For this review, use the dimensioned drawing (mm, ordinates from the lowest corner) and the shaded views. Round coordinates to 2 decimals unless told otherwise and drop trailing zeros. Order: outer loops, then holes, each group sorted by start corner. A loop starts at its lowest first (then second) coordinate and runs counter-clockwise, first axis right, second up. Notation, with made-up numbers: (84, -11) - (105, -11) arc R7 ccw to (105, -3) - close; hole circle Ø3 at (27.5, 76). An arc over 180 degrees is marked (long way). Write each question's results on one line, items separated by ' | '. Start each with the question number.
(1) Take a section at D-D, the plane y = 12.75. Give the boundary of the cut face in (x, z), plus the area to 3 significant figures.
(2) Take a section at B-B, the plane z = 27.5. Give the boundary of the cut face in (x, y).
(3) Take a section at A-A, the plane x = 28.5. Give the boundary of the cut face in (y, z), plus the area to 3 significant figures.
(4) For L1, parallel to X at y = 2.25, z = 28; L2, parallel to X at y = 10.75, z = 34; L3, parallel to Y at x = 28, z = 46, list the stretches that pass through material, from the lowest coordinate up. Write a range as from..to.
(5) Insertion check: pin 1 Ø9 at (x, y) = (28.5, 10) entering from +Z; pin 2 Ø2 at (x, y) = (43, 4) entering from -Z; pin 3 Ø1 at (y, z) = (6.5, 22) entering from -X; pin 4 Ø5 at (x, y) = (25.5, 18) entering from -Z. Each pin has a flat end and moves straight along its axis. Give the tip position at first contact, or say it passes through.
(6) Take a section at C-C, the plane y = 18. Give the boundary of the cut face in (x, z).
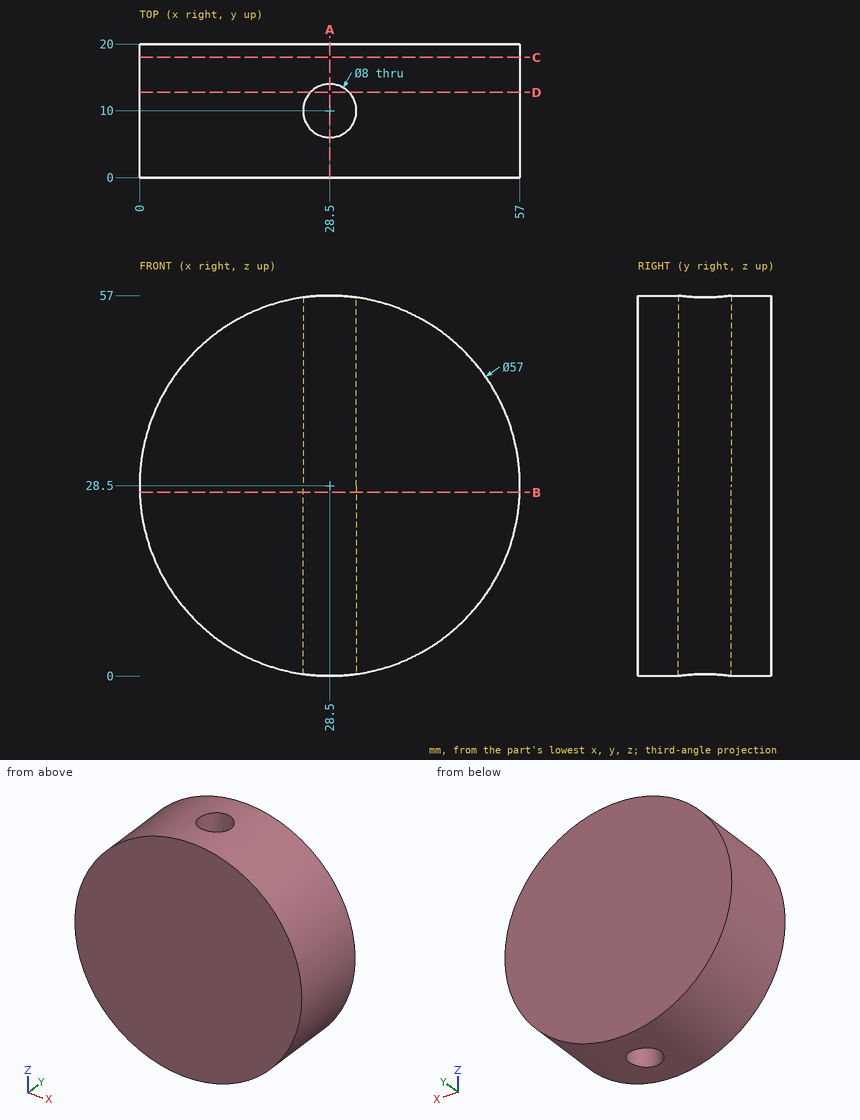
Results below:
1) outline: (25.6, 0.15) - (25.6, 56.85) arc R28.5 ccw to start; (31.4, 0.15) arc R28.5 ccw to (31.4, 56.85) - close | area: 2,220 mm^2
2) outline: (0.02, 0) - (56.98, 0) - (56.98, 20) - (0.02, 20) - close; hole circle Ø8 at (28.5, 10)
3) outline: (0, 0) - (6, 0) - (6, 57) - (0, 57) - close; (14, 0) - (20, 0) - (20, 57) - (14, 57) - close | area: 684 mm^2
4) L1: x = 0..57 | L2: x = 0.54..24.57, 32.43..56.46 | L3: y = 0..6.03, 13.97..20
5) pin 1: stops at z = 57 | pin 2: stops at z = 3.4 | pin 3: stops at x = 0.64 | pin 4: stops at z = 0
6) outline: circle Ø57 at (28.5, 28.5)
